The listing builds one solid part. Answer for the finished solid, in the listing's coordinates (mm). Face numbers are marked on the shaded views. A direction names the side the tool comes from. Give positions to 0.01 mm unless a question says otherwise; leave off trailing zeros. Write each loop counter-clockwise with the first axis right and the second up, starting at its lowest first coordinate (ties: lowest second). Pieces come first, ordered by that corner, then holes. Notation, with made-up numbers: (73, 58.5) - (101, 58.5) arc R24 ccw to (101, 73.5) - close; hole circle Ø6 at (-15, 76.5). An arc over 180 degrees is marked (long way). Return JSON: item names as keys, results as strings.
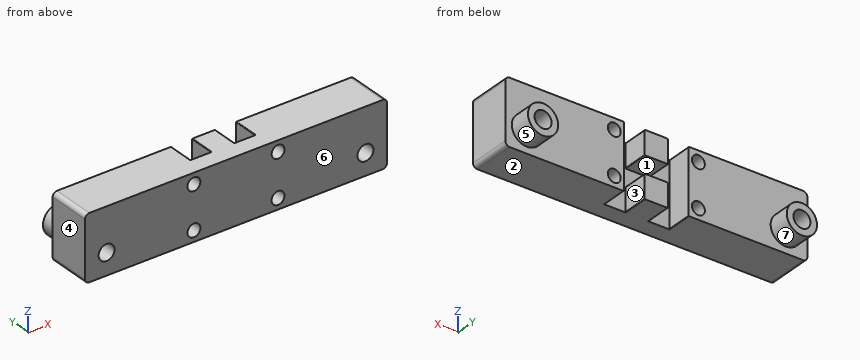
from build123d import *

# Parameters (mm, degrees)
SKETCH1_W           = 70
SKETCH1_H           = 15
SKETCH1_R           = 1.75
SKETCH1_R_2         = 1.5
BOSS_EXTRUDE1_DEPTH = 10
SKETCH2_W           = 15
SKETCH2_H           = 15
CUT_EXTRUDE1_DEPTH  = 6
SKETCH3_W           = 5.388877434
SKETCH3_H           = 5.5
BOSS_EXTRUDE2_DEPTH = 6
FILLET1_R           = 1
FILLET2_R           = 0.15
SKETCH4_R           = 3.5
SKETCH4_R_2         = 1.75
BOSS_EXTRUDE3_DEPTH = 5
SKETCH5_R           = 1.85
CUT_EXTRUDE2_DEPTH  = 74.143694192
SKETCH6_R           = 1.975
CUT_EXTRUDE3_DEPTH  = 4


with BuildPart() as part:
    # Sketch1 → Boss-Extrude1 (new body)
    with BuildSketch(Plane(origin=(0, 0, 0), x_dir=(1, 0, 0), z_dir=(0, 1, 0))):
        with Locations((35, 7.5)):
            Rectangle(SKETCH1_W, SKETCH1_H)
        with Locations(Location((5, 10, 0), (0, 0, 270))):
            Circle(SKETCH1_R, mode=Mode.SUBTRACT)
        with Locations(Location((65, 10, 0), (0, 0, 270))):
            Circle(SKETCH1_R, mode=Mode.SUBTRACT)
        with Locations(Location((25.25, 12.5, 0), (0, 0, 270))):
            Circle(SKETCH1_R_2, mode=Mode.SUBTRACT)
        with Locations(Location((44.75, 12.5, 0), (0, 0, 90))):
            Circle(SKETCH1_R_2, mode=Mode.SUBTRACT)
        with Locations(Location((44.75, 2.5, 0), (0, 0, 270))):
            Circle(SKETCH1_R_2, mode=Mode.SUBTRACT)
        with Locations(Location((25.25, 2.5, 0), (0, 0, 90))):
            Circle(SKETCH1_R_2, mode=Mode.SUBTRACT)
    extrude(amount=BOSS_EXTRUDE1_DEPTH)

    # Sketch2 → Cut-Extrude1 (cut)
    with BuildSketch(Plane(origin=(0, 10, 0), x_dir=(1, 0, 0), z_dir=(0, 1, 0))):
        with Locations((35, 7.5)):
            Rectangle(SKETCH2_W, SKETCH2_H)
    extrude(amount=-CUT_EXTRUDE1_DEPTH, mode=Mode.SUBTRACT)

    # Sketch3 → Boss-Extrude2 (add)
    with BuildSketch(Plane(origin=(0, 4, 0), x_dir=(1, 0, 0), z_dir=(0, 1, 0))):
        with Locations((35, 12.25)):
            Rectangle(SKETCH3_W, SKETCH3_H)
        with Locations((35, 2.75)):
            Rectangle(SKETCH3_W, SKETCH3_H)
    extrude(amount=BOSS_EXTRUDE2_DEPTH)

    # Fillet1
    fillet1_edges = [part.edges().sort_by_distance(p)[0] for p in [
        (0, 5, -15),
        (70, 5, -15),
        (70, 5, 0),
        (0, 5, 0),
    ]]
    fillet(fillet1_edges, radius=FILLET1_R)

    # Fillet2
    fillet2_edges = [part.edges().sort_by_distance(p)[0] for p in [
        (27.5, 7, 0),
        (27.5, 7, -15),
        (42.5, 7, -15),
        (42.5, 7, 0),
        (32.305561283, 7, -15),
        (32.305561283, 7, -9.5),
        (37.694438717, 7, -9.5),
        (37.694438717, 7, -15),
        (32.305561283, 7, 0),
        (37.694438717, 7, 0),
        (37.694438717, 7, -5.5),
    ]]
    fillet(fillet2_edges, radius=FILLET2_R)

    # Sketch4 → Boss-Extrude3 (add)
    # profile 1 of 2: a face of its own
    with BuildSketch(Plane(origin=(0, 10, 0), x_dir=(1, 0, 0), z_dir=(0, 1, 0))):
        with Locations(Location((5, 10, 0), (0, 0, 90))):
            Circle(SKETCH4_R)
        with Locations(Location((5, 10, 0), (0, 0, 90))):
            Circle(SKETCH4_R_2, mode=Mode.SUBTRACT)
    # profile 2 of 2: a face of its own
    with BuildSketch(Plane(origin=(0, 10, 0), x_dir=(1, 0, 0), z_dir=(0, 1, 0))):
        with Locations(Location((65, 10, 0), (0, 0, 90))):
            Circle(SKETCH4_R)
        with Locations(Location((65, 10, 0), (0, 0, 90))):
            Circle(SKETCH4_R_2, mode=Mode.SUBTRACT)
    extrude(amount=BOSS_EXTRUDE3_DEPTH)

    # Sketch5 → Cut-Extrude2 (cut, through all)
    with BuildSketch(Plane(origin=(0, 15, 0), x_dir=(1, 0, 0), z_dir=(0, 1, 0))):
        with Locations(Location((5, 10, 0), (0, 0, 270))):
            Circle(SKETCH5_R)
        with Locations(Location((65, 10, 0), (0, 0, 270))):
            Circle(SKETCH5_R)
    extrude(amount=-CUT_EXTRUDE2_DEPTH, mode=Mode.SUBTRACT)

    # Sketch6 → Cut-Extrude3 (cut)
    with BuildSketch(Plane(origin=(0, 15, 0), x_dir=(1, 0, 0), z_dir=(0, 1, 0))):
        with Locations(Location((5, 10, 0), (0, 0, 270))):
            Circle(SKETCH6_R)
        with Locations(Location((65, 10, 0), (0, 0, 270))):
            Circle(SKETCH6_R)
    extrude(amount=-CUT_EXTRUDE3_DEPTH, mode=Mode.SUBTRACT)


solid = part.part
Item 1: For the marked faces 1, 2 and 3, determine the directions among +Z, -Z, +X, -X, +Y, -Y from which every point of the face is accessible in a straight line to the end or side of a thin tool.
Answer below:
{"face 1": "+Y", "face 2": "-Z, +X, -X, +Y, -Y", "face 3": "+Z, -Z, +Y"}
Item 2: A cutting plane is placed at B-B on z = -2.5. Determine the outline of the cut face in (x, y).
Answer below:
{"outline": "(0, 0) - (23.75, 0) - (23.75, 10) - (0, 10) - close; (26.75, 0) - (43.25, 0) - (43.25, 10) - (42.5, 10) - (42.5, 4) - (37.69, 4) - (37.69, 10) - (32.31, 10) - (32.31, 4) - (27.5, 4) - (27.5, 10) - (26.75, 10) - close; (46.25, 0) - (70, 0) - (70, 10) - (46.25, 10) - close"}
Item 3: A cutting plane is placed at C-C on x = 44.75. Determine the outline of the cut face in (y, z).
Answer below:
{"outline": "(0, -15) - (10, -15) - (10, -14) - (0, -14) - close; (0, -11) - (10, -11) - (10, -4) - (0, -4) - close; (0, -1) - (10, -1) - (10, 0) - (0, 0) - close"}
Item 4: A flat-ended cylindrical pin translates along its axis: P1, Ø7.5, axis at x = 19.5, z = -9.5, coming from the +Y side. Find the tip coordinate at first contact, or state that the pin passes through.
Answer below:
{"P1": "stops at y = 10"}
Item 5: The mould has two halves that part along X. Classify the marked faces 4, 5, 6 and 7: +X half, -X half, draft (parallel to the pull), parting line (faces both ways), or undercut.
Answer below:
{"face 4": "-X half", "face 5": "undercut", "face 6": "draft", "face 7": "undercut"}
Item 6: Consider L1, parallel to X at y = 14.1, z = -10 (3 decimals); L2, parallel to X at y = 5.25, z = -2.5; L3, parallel to X at y = 2.5, z = -10. Determine where each line is inside the solid, lowest interval first.
Answer below:
{"L1": "x = 1.5 to 3.025, 6.975 to 8.5, 61.5 to 63.025, 66.975 to 68.5", "L2": "x = 0 to 23.75, 26.75 to 27.5, 32.31 to 37.69, 42.5 to 43.25, 46.25 to 70", "L3": "x = 0 to 3.15, 6.85 to 63.15, 66.85 to 70"}
Item 7: A cutting plane is placed at D-D on y = 9.25. Give the number of separate pieces and of enclosed holes in the cut face, then the cut area to 3 significant figures.
Answer below:
{"separate pieces": "4", "enclosed holes": "6", "area": "834 mm²"}
Item 8: A cutting plane is placed at A-A on x = 65. Determine the outline of the cut face in (y, z) (3 decimals), then the cut area to 4 significant figures.
Answer below:
{"outline": "(0, -15) - (10, -15) - (10, -13.5) - (15, -13.5) - (15, -11.975) - (11, -11.975) - (11, -11.85) - (0, -11.85) - close; (0, -8.15) - (11, -8.15) - (11, -8.025) - (15, -8.025) - (15, -6.5) - (10, -6.5) - (10, 0) - (0, 0) - close", "area": "128.5 mm²"}
